```python
from build123d import *

# Parameters (mm, degrees)
F0_R     = 3.175
F1_DEPTH = 19.05
F2_R     = 4.7879
F3_DEPTH = 50.8
F5_DEPTH = 279.4


# Not quite as in the source:
# - a feature names something its author has since deleted; it is built from what else it names


with BuildPart() as f1:
    # F0 (on Top) → F1 (new body)
    with BuildSketch(Plane.XY):
        with BuildLine():
            Line((-118.9269337424, 53.8231658584), (-147.8829337424, 53.8231658584))
            Line((-147.8829337424, 53.8231658584), (-147.8829337424, -16.0268341416))
            Line((-147.8829337424, -16.0268341416), (-147.8829337424, -19.2018341416))
            Line((-147.8829337424, -19.2018341416), (-135.1829337424, -19.2018341416))
            Line((-135.1829337424, -19.2018341416), (-135.1829337424, -130.3268341416))
            Line((-135.1829337424, -130.3268341416), (-147.8829337424, -130.3268341416))
            Line((-147.8829337424, -130.3268341416), (-147.8829337424, -136.6768341416))
            Line((-147.8829337424, -136.6768341416), (-147.8829337424, -171.6018341416))
            Line((-147.8829337424, -171.6018341416), (-147.8829337424, -203.3518341416))
            Line((-147.8829337424, -203.3518341416), (-118.9269337424, -203.3518341416))
            ThreePointArc((-118.9269337424, -203.3518341416), (-116.6818697121, -204.2817701113), (-115.7519337424, -206.5268341416))
            Line((-115.7519337424, -206.5268341416), (-115.7519337424, -245.9476341416))
            ThreePointArc((-115.7519337424, -245.9476341416), (-113.8920618029, -250.4377622021), (-109.4019337424, -252.2976341416))
            Line((-109.4019337424, -252.2976341416), (-74.8579337424, -252.2976341416))
            ThreePointArc((-74.8579337424, -252.2976341416), (-70.3678056819, -250.4377622021), (-68.5079337424, -245.9476341416))
            Line((-68.5079337424, -245.9476341416), (-68.5079337424, -203.3518341416))
            Line((-68.5079337424, -203.3518341416), (-55.8079337424, -203.3518341416))
            Line((-55.8079337424, -203.3518341416), (-55.8079337424, -184.3018341416))
            Line((-55.8079337424, -184.3018341416), (-5.0079337424, -184.3018341416))
            Line((-5.0079337424, -184.3018341416), (-5.0079337424, -171.6018341416))
            Line((-5.0079337424, -171.6018341416), (77.5420662576, -171.6018341416))
            Line((77.5420662576, -171.6018341416), (77.5420662576, -146.2018341416))
            Line((77.5420662576, -146.2018341416), (-5.0079337424, -146.2018341416))
            Line((-5.0079337424, -146.2018341416), (-5.0079337424, -133.5018341416))
            Line((-5.0079337424, -133.5018341416), (-27.2329337424, -133.5018341416))
            Line((-27.2329337424, -133.5018341416), (-116.1329337424, -133.5018341416))
            Line((-116.1329337424, -133.5018341416), (-116.1329337424, -16.0268341416))
            Line((-116.1329337424, -16.0268341416), (-22.9684459845, -16.0268341416))
            Line((-22.9684459845, -16.0268341416), (-5.0079337424, -16.0268341416))
            Line((-5.0079337424, -16.0268341416), (-5.0079337424, -7.9982466186))
            Line((-5.0079337424, -7.9982466186), (-5.0079337424, 15.7231658584))
            Line((-5.0079337424, 15.7231658584), (77.5420662576, 15.7231658584))
            Line((77.5420662576, 15.7231658584), (77.5420662576, 41.1231658584))
            Line((77.5420662576, 41.1231658584), (-5.0079337424, 41.1231658584))
            Line((-5.0079337424, 41.1231658584), (-5.0079337424, 53.8231658584))
            Line((-5.0079337424, 53.8231658584), (-65.3329337424, 53.8231658584))
            ThreePointArc((-65.3329337424, 53.8231658584), (-67.5779977727, 54.7531018282), (-68.5079337424, 56.9981658584))
            Line((-68.5079337424, 56.9981658584), (-68.5079337424, 115.4689658584))
            ThreePointArc((-68.5079337424, 115.4689658584), (-70.3678056819, 119.959093919), (-74.8579337424, 121.8189658584))
            Line((-74.8579337424, 121.8189658584), (-109.4019337424, 121.8189658584))
            ThreePointArc((-109.4019337424, 121.8189658584), (-113.8920618029, 119.959093919), (-115.7519337424, 115.4689658584))
            Line((-115.7519337424, 115.4689658584), (-115.7519337424, 56.9981658584))
            ThreePointArc((-115.7519337424, 56.9981658584), (-116.6818697121, 54.7531018282), (-118.9269337424, 53.8231658584))
        make_face()
        with Locations((-138.3579337424, -193.8268341416)):
            Circle(F0_R, mode=Mode.SUBTRACT)
        with Locations((-65.3329337424, -193.8268341416)):
            Circle(F0_R, mode=Mode.SUBTRACT)
        with Locations((-46.2829337424, -158.9018341416)):
            Circle(F0_R, mode=Mode.SUBTRACT)
        with Locations((4.5170662576, -158.9018341416)):
            Circle(F0_R, mode=Mode.SUBTRACT)
        with Locations((55.3170662576, -158.9018341416)):
            Circle(F0_R, mode=Mode.SUBTRACT)
        with Locations((-138.3579337424, -6.5018341416)):
            Circle(F0_R, mode=Mode.SUBTRACT)
        with Locations((-65.3329337424, -6.5018341416)):
            Circle(F0_R, mode=Mode.SUBTRACT)
        with Locations((-46.2829337424, 28.4231658584)):
            Circle(F0_R, mode=Mode.SUBTRACT)
        with Locations((4.5170662576, 28.4231658584)):
            Circle(F0_R, mode=Mode.SUBTRACT)
        with Locations((55.3170662576, 28.4231658584)):
            Circle(F0_R, mode=Mode.SUBTRACT)
    extrude(amount=F1_DEPTH)

    # F2 (on face) → F3 (cut)
    with BuildSketch(Plane(origin=(-147.8829337424, 0, 0), x_dir=(0, -1, 0), z_dir=(-1, 0, 0))):
        with Locations((103.9362341416, 15.875)):
            Circle(F2_R)
    extrude(amount=-F3_DEPTH, mode=Mode.SUBTRACT)

    # F4 (on face) → F5 (cut)
    with BuildSketch(Plane.XZ.offset(203.3518341416)):
        Polygon((-120.3866271722, 0), (-147.8829337424, 15.875), (-147.8829337424, 0), align=None)
    extrude(amount=-F5_DEPTH, mode=Mode.SUBTRACT)


solid = f1.part
```
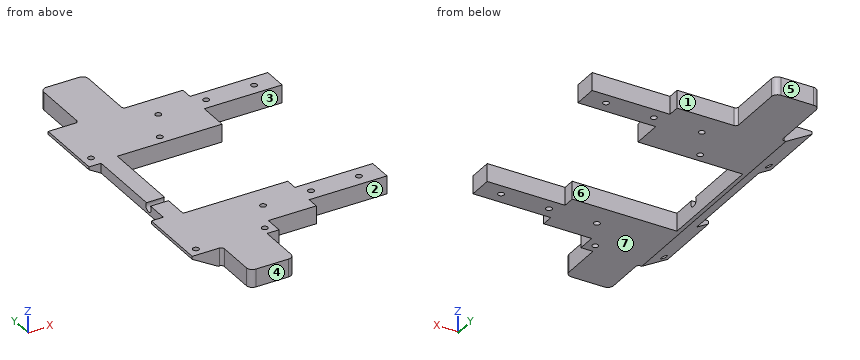
Can you work these out from the model? Positions are in its coordinate system, mm. Face numbers are marked on the shaded views. A direction names the side the tool comes from. Give positions to 0.01 mm unless a question says otherwise; leave off trailing zeros. Order: outer loops, then holes, each group sorted by start corner. A loop starts at its lowest first (then second) coordinate and runs counter-clockwise, first axis right, second up. Notation, with made-up numbers: M 43.5,-26.5 L 53.5,-26.5 A20 ccw 53.5,-11.5 Z; hole C 56,-1 d9. An arc over 180 degrees is marked long. Write item = value, one per line. Start each with the question number.
Q1. Suppose I cut it at C-C (x = -130.5). Write out the boundary of the cut face in (y, z) (3 decimals), plus the area to 3 significant figures.
Q2. We'd pull the mould along Y, two halves only. Please class the marked faces 5, 6 and 7: pulls with the +Y half, pulls with the -Y half, needs draft (parallel to the pull), parting line crosses it, or undercut.
Q3. For the marked faces 1, 2, 3 and 4, which set-ups out of +Z, -Z, +X, -X, +Y, -Y let a thin tool reach every point of the face, with its end or its side?
Q4. Will these pins go through, and if not, where does the flat tip stop? pin 1 Ø2 at (x, z) = (19, 7.5) entering from +Y; pin 2 Ø9.5 at (y, z) = (-6, 10) entering from +X; pin 3 Ø1.5 at (y, z) = (-145, 3) entering from -X.
Q5. I need wall thicknesses on probe 1 along Y at (x, z) = (-58, 13); probe 2 along Y at (x, z) = (-80.5, 14); probe 3 along X at (y, z) = (-6, 13.5). Which ranges of each line are inside material? Lowest first, please. Write a range as [from, to].
Q6. Suppose I cut it at B-B (y = -140). Write out the boundary of the cut face in (x, z) (3 decimals), plus the area to 3 significant figures.
Q7. Suppose I cut it at A-A (x = 36). Write out the boundary of the cut face in (y, z), plus the area to 3 significant figures.
Q8. Suppose I cut it at D-D (y = -42.5). Write out the boundary of the cut face in (x, z).
Check result:
q1.outline = M -203.352,5.839 L 53.823,5.839 L 53.823,19.05 L -100.352,19.05 A4.788 cw long -107.52,19.05 L -203.352,19.05 Z
q1.area = 3,330 mm2
q2.face_5 = pulls with the +Y half
q2.face_6 = undercut
q2.face_7 = needs draft
q3.face_1 = +Z, -Z, +X, +Y
q3.face_2 = +Z, -Z, +X, -Y
q3.face_3 = +Z, -Z, +X
q3.face_4 = +Z, -Z, +X, -X, -Y
q4.pin_1 = 41.12
q4.pin_2 = -5.01
q4.pin_3 = -126.88
q5.probe_1 = [-203.35, -133.5], [-16.03, 53.82]
q5.probe_2 = [-252.3, -133.5], [-16.03, 121.82]
q5.probe_3 = [-143.77, -141.49], [-135.22, -68.47], [-62.2, -5.01]
q6.outline = M -147.883,15.875 L -120.387,0 L -5.008,0 L -5.008,19.05 L -147.883,19.05 Z
q6.area = 2,500 mm2
q7.outline = M -171.6,0 L -146.2,0 L -146.2,19.05 L -171.6,19.05 Z; M 15.72,0 L 41.12,0 L 41.12,19.05 L 15.72,19.05 Z
q7.area = 968 mm2
q8.outline = M -135.18,8.54 L -120.39,0 L -116.13,0 L -116.13,19.05 L -135.18,19.05 Z
